```python
from build123d import *

# Parameters (mm, degrees)
F1_DEPTH = 100
F2_W     = 20
F2_H     = 87
F4_W     = 10.5
F4_H     = 48.8


with BuildPart() as f1:
    # F0 (on Front) → F1 (new body)
    with BuildSketch(Plane.XZ):
        Polygon((-50, 0), (0, 0), (0, 40), (-13.2016703318, 40), (-16.5485225135, 20), (-50, 20), align=None)
    extrude(amount=F1_DEPTH)

    # F2 (on face) → F5 section 0
    with BuildSketch(Plane.XY.offset(20)):
        with Locations((-36.5485225135, -50)):
            Rectangle(F2_W, F2_H)
    # F4 (on offset) → F5 section 1
    with BuildSketch(Plane.XY.offset(65)):
        with Locations((-31.7985225135, -50)):
            Rectangle(F4_W, F4_H)
    loft()


solid = f1.part
```
Check sheet for the modelled part. Datum: model origin and axes. Units: mm. A direction names the side the tool comes from. Give positions to 0.01 mm unless a question says otherwise; leave off trailing zeros. Write each loop counter-clockwise with the first axis right and the second up, starting at its lowest first coordinate (ties: lowest second). Pieces come first, ordered by that corner, then holes.
Item 1: Draft check along X on faces 4 (the face through (-50, -49, 10)), 5 (the face through (-25, -49, 0)), 6 (the face through (-26, -49, 20)). Enter one of: released by +X, released by -X, zero draft, split by the parting line, or undercut.
Item 2: Cross-section at A-A (x = -18). Enter the section's corners in (y, z), and give its area (3 significant figures).
Item 3: Cross-section at B-B (x = -11). Enter the section's corners in (y, z), and give its area (3 significant figures).
Item 4: Access from +Z, -Z, +X, -X, +Y, -Y to the whole of each face (thin tool, end or side, straight path). Record for faces 1 (the face through (-7, -49, 40)), 2 (the face through (-14.85, -49.3, 30.14)), 3 (the face through (-20, -100, 16)).
Item 5: Scan lines: L1, parallel to X at y = -88.5, z = 26; L2, parallel to Z at x = -17, y = -21; L3, parallel to Z at x = -9, y = -6. Record each from-to range of solid material in increasing order.
Item 6: Gauge pin test, flat ends, axial feed: pin 1 (2 mm diameter, centred on y = -44, z = 44.5, fed in from -X); pin 2 (12 mm diameter, centred on x = -23, z = 26.5, fed in from +Y); pin 3 (6 mm diameter, centred on x = -39, z = 50.5, fed in from +Y). Record the tip position at first contact, or that the pin passes through.
Report:
1. face 4: released by -X
1. face 5: zero draft
1. face 6: undercut
2. outline: (-100, 0) - (0, 0) - (0, 20) - (-100, 20) - close
2. area: 2,000 mm2
3. outline: (-100, 0) - (0, 0) - (0, 40) - (-100, 40) - close
3. area: 4,000 mm2
4. face 1: +Z, +X, +Y, -Y
4. face 2: +Z, +Y, -Y
4. face 3: +Z, -Z, +X, -X, -Y
5. L1: x = -45.28 to -26.55, -15.54 to 0
5. L2: z = 0 to 20
5. L3: z = 0 to 40
6. pin 1: stops at x = -41.59
6. pin 2: stops at y = -7.21
6. pin 3: stops at y = -18.17
